Geometry check sheet. Reference: the model listing, model coordinates, mm. Face numbers are marked on the shaded views. Give positions to 0.01 mm unless a question says otherwise; leave off trailing zeros. Loops run counter-clockwise (first coordinate to the right, second up) from the corner with the lowest first, then second, coordinate; pieces in that order, holes last. Notation, with made-up numbers: (38.25, 29) -> (66.25, 29) arc R21 cw to (66.25, 49) -> close; hole circle Ø5 at (-39, 23.5). An arc over 180 degrees is marked (long way). One line per item, written item: value. Start each with the question number.
(1) Gauge pin test, flat ends, axial feed: pin 1 Ø6 at (x, y) = (110.5, -6.5) entering from -Z; pin 2 Ø8 at (x, y) = (53.5, -4) entering from -Z; pin 3 Ø5 at (x, z) = (43, -3) entering from +Y; pin 4 Ø1 at (x, y) = (82.5, 7) entering from -Z. Record the tip position at first contact, or that the pin passes through.
(2) Scan lines: line 1 along Y through (x, z) = (66, 0); line 2 along Z through (x, y) = (135, 2.5); line 3 along Y through (x, z) = (9, 7.25). Record each from-to range of solid material in increasing order. Write a range as from..to.
(3) Sectioned sample at A-A, the plane z = 0. Record the cut outline in (x, y).
(4) Sectioned sample at C-C, the plane x = 77. Record the cut outline in (y, z), then the cut area to 3 significant figures.
(5) Draft check along Z on the marked faces 1 and 2. Enter one of: pulls with the +Z half, pulls with the -Z half, needs draft (parallel to the pull), parting line crosses it, or undercut.
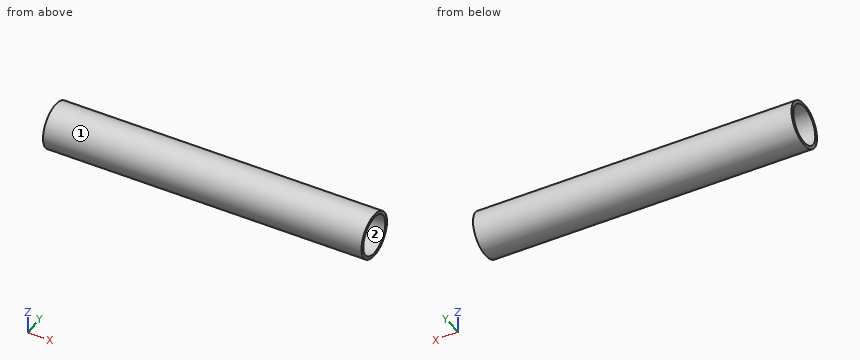
from build123d import *

# Parameters (mm, degrees)
CYLINDER001_R     = 9.5
CYLINDER001_DEPTH = 156
CYLINDER_R        = 11
CYLINDER_DEPTH    = 156
CUT_PITCH_ANGLE   = 90


with BuildPart() as int:
    # Cylinder001 → Cylinder001 (new body)
    with BuildSketch(Plane.XY):
        Circle(CYLINDER001_R)
    extrude(amount=CYLINDER001_DEPTH)


with BuildPart() as steeltube:
    # Cylinder → Cylinder (new body)
    with BuildSketch(Plane.XY):
        Circle(CYLINDER_R)
    extrude(amount=CYLINDER_DEPTH)

    # Cut: cut INT
    add(int.part, mode=Mode.SUBTRACT)


with BuildPart() as steeltube_1:
    # Cut pitch: moved
    add(steeltube.part.rotate(Axis((0, 0, 0), (0, 1, 0)), CUT_PITCH_ANGLE))


with BuildPart() as steeltube_2:
    # Cut placement: moved
    add(steeltube_1.part)


solid = steeltube_2.part
Calculated:
1. pin 1: stops at z = -10.43
1. pin 2: stops at z = -11
1. pin 3: stops at y = 10.99
1. pin 4: stops at z = -8.87
2. line 1: y = -11..-9.5, 9.5..11
2. line 2: z = -10.71..-9.17, 9.17..10.71
2. line 3: y = -8.27..-6.14, 6.14..8.27
3. outline: (0, -11) -> (156, -11) -> (156, -9.5) -> (0, -9.5) -> close; (0, 9.5) -> (156, 9.5) -> (156, 11) -> (0, 11) -> close
4. outline: circle Ø22 at (0, 0); hole circle Ø19 at (0, 0)
4. area: 96.6 mm2
5. face 1: parting line crosses it
5. face 2: undercut
